Input: part model. Units: mm. Frame: model coordinates. A direction names the side the tool comes from. Coordinates: 2 decimals unless noted, no trailing zeros. Write each loop counter-clockwise with the first axis right and the second up, starting at its lowest first coordinate (ties: lowest second). Pieces come first, ordered by that corner, then holes.
1) Pin query (flat end, axial travel): pin 1 Ø11 at (y, z) = (7, -5.5) entering from +X; pin 2 Ø12 at (y, z) = (15.5, -8) entering from -X; pin 3 Ø2 at (x, y) = (109, -19) entering from +Z. Return the tip coordinate at first contact, or that it passes through.
2) Set-up query: faces 4 (the flat face through (38, 16.825, -23)), 5 (the cylindrical face through (110.1, -0.3, -26.9)), 6 (the flat face through (49, -20, 0)), 7 (the cylindrical face through (49, 0, -35)), 8 (the flat face through (49, -15, -2)). Return all of +Z, -Z, +X, -X, +Y, -Y with unobstructed straight access to the full face (end or side cutting, diameter ignored); none if empty.
3) Section query A-A (y = 0). Output: boundary loops of the cut face in (x, z), then the cut area to 3 significant figures.
4) Section query D-D (x = -2.5). Output: boundary loops of the cut face in (y, z).
5) Section query B-B (z = 8). Output: boundary loops of the cut face in (x, y) (3 decimals), then the cut area to 3 significant figures.
6) Line query: L1, parallel to Y at x = 97, z = 0 (3 decimals); L2, parallel to X at y = 5, z = -22; L3, parallel to X at y = 14, z = -13. Output: solid intervals per line, ascending.
7) Draft query along X for faces 1 (the flat face through (0, 18, -24)), 2 (the flat face through (-10, 0, -20)), 3 (the flat face through (0, -1, -5)). Return one class per face: pulls with the +X half, pulls with the -X half, needs draft (parallel to the pull), parting line crosses it, or undercut.
from build123d import *

# Parameters (mm, degrees)
BOSS_EXTRUDE1_DEPTH = 100
SHELL3_START        = 5
SHELL3_DEPTH        = 90
BOSS_EXTRUDE2_DEPTH = 20
SKETCH7_W           = 100
SKETCH7_H           = 50.81
CUT_EXTRUDE6_DEPTH  = 3.175
CUT_EXTRUDE1_REACH  = 130.062
SKETCH2_R           = 0.8
SKETCH2_R_2         = 3
SKETCH8_R           = 1
CUT_EXTRUDE7_DEPTH  = 3
CUT_EXTRUDE8_DEPTH  = 20


# Read off the part's stored shape, not the designer's step: Shell3
with BuildPart() as part:
    # Sketch1 → Boss-Extrude1 (new body)
    with BuildSketch(Plane(origin=(0, 0, 0), x_dir=(0, 0, -1), z_dir=(1, 0, 0))):
        with BuildLine():
            Line((-20, 20), (20, 20))
            ThreePointArc((20, 20), (40, 0), (20, -20))
            Line((20, -20), (-20, -20))
            Line((-20, -20), (-20, 20))
        make_face()
    extrude(amount=BOSS_EXTRUDE1_DEPTH)

    # Shell3 outline → Shell3 (cut)
    with BuildSketch(Plane.YZ.offset(SHELL3_START)):
        with BuildLine():
            Line((15, -20), (20, -20))
            Line((20, -20), (20, 15))
            Line((20, 15), (-15, 15))
            Line((-15, 15), (-15, -20))
            ThreePointArc((-15, -20), (0, -35), (15, -20))
        make_face()
    extrude(amount=SHELL3_DEPTH, mode=Mode.SUBTRACT)

    # Sketch9 → Boss-Extrude2 (add)
    with BuildSketch(Plane(origin=(100, 0, 0), x_dir=(0, 0, -1), z_dir=(1, 0, 0))):
        with BuildLine():
            Line((20, 20), (20, -20))
            ThreePointArc((20, -20), (40, 0), (20, 20))
        make_face()
    boss_extrude2 = extrude(amount=BOSS_EXTRUDE2_DEPTH)

    # Mirror1: Boss-Extrude2 across plane
    add(boss_extrude2.mirror(Plane(origin=(50, 0, 0), x_dir=(0, 0, 1), z_dir=(1, 0, 0))))

    # Sketch7 → Cut-Extrude6 (cut)
    with BuildSketch(Plane(origin=(0, 20, 0), x_dir=(1, 0, 0), z_dir=(0, 1, 0))):
        with Locations((50, 5.405)):
            Rectangle(SKETCH7_W, SKETCH7_H)
    extrude(amount=-CUT_EXTRUDE6_DEPTH, mode=Mode.SUBTRACT)

    # Cut-Extrude1: up to this face of the body (flat: up to its plane)
    cut_extrude1_end = Plane(part.part.faces().sort_by_distance((0, -1.5875, 0))[0])
    # Sketch2 → Cut-Extrude1 (cut, up to the picked face)
    with BuildSketch(Plane(origin=(100, 0, 0), x_dir=(0, 0, -1), z_dir=(1, 0, 0)), mode=Mode.PRIVATE) as cut_extrude1_sk1:
        with Locations(Location((0, -5.25, 0), (0, 0, 180))):
            Circle(SKETCH2_R)
    cut_extrude1_tool1 = split(extrude(cut_extrude1_sk1.sketch, amount=-CUT_EXTRUDE1_REACH, mode=Mode.PRIVATE), bisect_by=cut_extrude1_end, keep=Keep.BOTH, mode=Mode.PRIVATE)
    # Sketch2 → Cut-Extrude1 (cut, up to the picked face)
    with BuildSketch(Plane(origin=(100, 0, 0), x_dir=(0, 0, -1), z_dir=(1, 0, 0)), mode=Mode.PRIVATE) as cut_extrude1_sk2:
        with Locations(Location((0, 0, 0), (0, 0, 180))):
            Circle(SKETCH2_R_2)
    cut_extrude1_tool2 = split(extrude(cut_extrude1_sk2.sketch, amount=-CUT_EXTRUDE1_REACH, mode=Mode.PRIVATE), bisect_by=cut_extrude1_end, keep=Keep.BOTH, mode=Mode.PRIVATE)
    # Sketch2 → Cut-Extrude1 (cut, up to the picked face)
    with BuildSketch(Plane(origin=(100, 0, 0), x_dir=(0, 0, -1), z_dir=(1, 0, 0)), mode=Mode.PRIVATE) as cut_extrude1_sk3:
        with Locations(Location((0, 5.25, 0), (0, 0, 180))):
            Circle(SKETCH2_R)
    cut_extrude1_tool3 = split(extrude(cut_extrude1_sk3.sketch, amount=-CUT_EXTRUDE1_REACH, mode=Mode.PRIVATE), bisect_by=cut_extrude1_end, keep=Keep.BOTH, mode=Mode.PRIVATE)
    add(cut_extrude1_tool1.solids().sort_by(Axis((100, -5.25, 0), (-1, 0, 0)))[0], mode=Mode.SUBTRACT)
    add(cut_extrude1_tool2.solids().sort_by(Axis((100, 0, 0), (-1, 0, 0)))[0], mode=Mode.SUBTRACT)
    add(cut_extrude1_tool3.solids().sort_by(Axis((100, 5.25, 0), (-1, 0, 0)))[0], mode=Mode.SUBTRACT)

    # Sketch8 → Cut-Extrude7 (cut)
    with BuildSketch(Plane(origin=(0, 16.825, 0), x_dir=(1, 0, 0), z_dir=(0, 1, 0))):
        with Locations(Location((97.5, -17.5, 0), (0, 0, 270))):
            Circle(SKETCH8_R)
        with Locations(Location((97.5, 18.31, 0), (0, 0, 270))):
            Circle(SKETCH8_R)
        with Locations(Location((2.5, -17.5, 0), (0, 0, 90))):
            Circle(SKETCH8_R)
        with Locations(Location((2.5, 18.31, 0), (0, 0, 90))):
            Circle(SKETCH8_R)
    extrude(amount=-CUT_EXTRUDE7_DEPTH, mode=Mode.SUBTRACT)

    # Sketch10 → Cut-Extrude8 (cut)
    with BuildSketch(Plane(origin=(120, 0, 0), x_dir=(0, 0, -1), z_dir=(1, 0, 0))):
        with BuildLine():
            Line((20, 17.989163405), (20, -17.989163405))
            ThreePointArc((20, -17.989163405), (26.9, 0), (20, 17.989163405))
        make_face()
    extrude(amount=-CUT_EXTRUDE8_DEPTH, mode=Mode.SUBTRACT)


solid = part.part
Answer:
1. pin 1: stops at x = 100
1. pin 2: stops at x = 0
1. pin 3: stops at z = -20
2. face 4: +Z, -Z, +Y
2. face 5: +Z, +X
2. face 6: +Z, -Z, +X, -X, -Y
2. face 7: none
2. face 8: +Y
3. outline: (-20, -40) - (120, -40) - (120, -26.9) - (100, -26.9) - (100, -3) - (95, -3) - (95, -35) - (5, -35) - (5, -3) - (0, -3) - (0, -20) - (-20, -20) - close; (0, 3) - (5, 3) - (5, 15) - (95, 15) - (95, 3) - (100, 3) - (100, 20) - (0, 20) - close
3. area: 2,100 mm2
4. outline: (-20, -20) arc R20 ccw to (20, -20) - close
5. outline: (0, -20) - (100, -20) - (100, 16.825) - (95, 16.825) - (95, -15) - (5, -15) - (5, 16.825) - (0, 16.825) - close
5. area: 818 mm2
6. L1: y = -20 to -6.05, -4.45 to -3, 3 to 4.45, 6.05 to 16.825
6. L2: x = -20 to 5, 95 to 100
6. L3: x = 0 to 5, 95 to 100
7. face 1: undercut
7. face 2: needs draft
7. face 3: pulls with the -X half
